from build123d import *


with BuildPart() as part:
    # Sketch1 → Revolve1 (revolve)
    with BuildSketch(Plane.XY, mode=Mode.PRIVATE) as revolve1_sk:
        with BuildLine():
            Line((-40, 20), (-50, 20))
            Line((-50, 20), (-50, 0))
            Line((-50, 0), (0, 0))
            Line((0, 0), (0, 12.26993865))
            Line((0, 12.26993865), (29.439071242, 12.26993865))
            Line((29.439071242, 12.26993865), (29.439071242, 28.82661238))
            Line((29.439071242, 28.82661238), (26.939071242, 28.82661238))
            Line((26.939071242, 28.82661238), (26.939071242, 70.956055766))
            ThreePointArc((26.939071242, 70.956055766), (25.684040418, 70.638264837), (24.439071242, 70.283095588))
            Line((24.439071242, 70.283095588), (24.439071242, 28.82661238))
            Line((24.439071242, 28.82661238), (19.439071242, 28.82661238))
            Line((19.439071242, 28.82661238), (19.439071242, 68.432672522))
            ThreePointArc((19.439071242, 68.432672522), (18.179445476, 67.85181502), (16.939071242, 67.230909015))
            Line((16.939071242, 67.230909015), (16.939071242, 28.82661238))
            Line((16.939071242, 28.82661238), (11.939071242, 28.82661238))
            Line((11.939071242, 28.82661238), (11.939071242, 64.18039577))
            ThreePointArc((11.939071242, 64.18039577), (10.671746733, 63.249245387), (9.439071242, 62.272688383))
            Line((9.439071242, 62.272688383), (9.439071242, 28.82661238))
            Line((9.439071242, 28.82661238), (4.439071242, 28.82661238))
            Line((4.439071242, 28.82661238), (4.439071242, 52.883509313))
            Line((4.439071242, 52.883509313), (-10.560928758, 52.883509313))
            Line((-10.560928758, 52.883509313), (-25.483605064, 42.81803705))
            Line((-25.483605064, 42.81803705), (-25.483605064, 26.193767786))
            Line((-25.483605064, 26.193767786), (-25.483605064, 21.51803705))
            Line((-25.483605064, 21.51803705), (-25.483605064, 21.193767786))
            Line((-25.483605064, 21.193767786), (-25.483605064, 20))
            ThreePointArc((-25.483605064, 20), (-28.412537252, 12.928932188), (-35.483605064, 10))
            Line((-35.483605064, 10), (-40, 10))
            Line((-40, 10), (-40, 20))
        make_face()
        with BuildLine():
            Line((29.439071242, 28.82661238), (29.439071242, 12.26993865))
            Line((29.439071242, 12.26993865), (44.439071242, 12.26993865))
            Line((44.439071242, 12.26993865), (44.439071242, 28.82661238))
            Line((44.439071242, 28.82661238), (41.939071242, 28.82661238))
            Line((41.939071242, 28.82661238), (41.939071242, 71.836959972))
            ThreePointArc((41.939071242, 71.836959972), (40.690646644, 71.963785236), (39.439071242, 72.054381233))
            Line((39.439071242, 72.054381233), (39.439071242, 28.82661238))
            Line((39.439071242, 28.82661238), (34.439071242, 28.82661238))
            Line((34.439071242, 28.82661238), (34.439071242, 72.054381233))
            ThreePointArc((34.439071242, 72.054381233), (33.187495839, 71.963785236), (31.939071242, 71.836959972))
            Line((31.939071242, 71.836959972), (31.939071242, 28.82661238))
            Line((31.939071242, 28.82661238), (29.439071242, 28.82661238))
        make_face()
        with BuildLine():
            Line((44.439071242, 28.82661238), (44.439071242, 12.26993865))
            Line((44.439071242, 12.26993865), (100, 12.26993865))
            Line((100, 12.26993865), (100, 27.26993865))
            Line((100, 27.26993865), (80, 27.26993865))
            Line((80, 27.26993865), (80, 48.56993865))
            Line((80, 48.56993865), (70, 48.56993865))
            Line((70, 48.56993865), (70, 28.82661238))
            Line((70, 28.82661238), (65, 28.82661238))
            Line((65, 28.82661238), (65, 61.803487266))
            ThreePointArc((65, 61.803487266), (63.768152096, 62.813233579), (62.5, 63.776990361))
            Line((62.5, 63.776990361), (62.5, 28.82661238))
            Line((62.5, 28.82661238), (56.939071242, 28.82661238))
            Line((56.939071242, 28.82661238), (56.939071242, 67.230909015))
            ThreePointArc((56.939071242, 67.230909015), (55.698697008, 67.85181502), (54.439071242, 68.432672522))
            Line((54.439071242, 68.432672522), (54.439071242, 28.82661238))
            Line((54.439071242, 28.82661238), (49.439071242, 28.82661238))
            Line((49.439071242, 28.82661238), (49.439071242, 70.283095588))
            ThreePointArc((49.439071242, 70.283095588), (48.194102066, 70.638264837), (46.939071242, 70.956055766))
            Line((46.939071242, 70.956055766), (46.939071242, 28.82661238))
            Line((46.939071242, 28.82661238), (44.439071242, 28.82661238))
        make_face()
    revolve(revolve1_sk.sketch.rotate(Axis((-50, -15, 0), (1, 0, 0)), 180), axis=Axis((-50, -15, 0), (1, 0, 0)))


solid = part.part
Can you work these out from the model? Positions are in its coordinate system, mm. A direction names the side the tool comes from. Coordinates: 2 decimals unless noted, no trailing zeros. Order: outer loops, then holes, each group sorted by start corner. A loop starts at its lowest first (then second) coordinate and runs counter-clockwise, first axis right, second up. Notation, with made-up numbers: (87.5, 87.5) - (114.5, 87.5) arc R14 ccw to (114.5, 94.5) - close; hole circle Ø5 at (86.5, 79.5). An arc over 180 degrees is marked (long way). Answer as a JSON object with one key per item and string values. Group by question number.
Q1. Imagine slicing it at A-A (x = -3). Please give me the cut outline in (y, z), and give its area (3 significant figures).
Q2. Imagine slicing it at D-D (x = 22). Please give me the cut outline in (y, z), and give its area (3 significant figures).
Q3. I need wall thicknesses on line 1 (X direction, y = -92.5, z = -22.5); line 2 (Z direction, x = -36.5, y = -15); line 3 (Z direction, x = -17, y = -15). Which ranges of each line are inside material? Lowest first, please. Write a range as from..to.
Q4. Will these pins go through, and if not, where does the flat tip stop? P1, Ø10, axis at y = 32.5, z = 18, coming from the -X side; P2, Ø6, axis at x = -12, y = 25.5, coming from the +Z side; P3, Ø12, axis at x = 63, z = -51, coming from the +Y side.
Q5. We'd pull the mould along X, two halves only. Please class faces 1 (the face through (80, -2, 41)), 2 (the face through (4.439, -16, 44)), 3 (the face through (-50, -30, 7)): +X half, -X half, draft (parallel to the pull), parting line (faces both ways), or undercut.
Q6. Imagine slicing it at B-B (z = -72). Give the number of separate pieces and of enclosed holes in the cut face, and give its area (3 significant figures).
Q7. On a 3-axis mill with a long thin cutter (end or side, diameter ignored), from which of +Z, -Z, +X, -X, +Y, -Y can I reach the whole of each face in a straight line? I mean faces 4 (the face through (50.7, -11.45, -27.038)), 5 (the face through (-45.07, -7.413, 34.168)), 6 (the face through (21.904, -9.295, -43.454)), 7 (the face through (-24.65, -0.015, -0.66)). Say none if no direction works.
Determined:
{
 "1": {"outline": "circle Ø135.77 at (-15, 0); hole circle Ø30 at (-15, 0)", "area": "13,800 mm2"},
 "2": {"outline": "circle Ø87.65 at (-15, 0); hole circle Ø54.54 at (-15, 0)", "area": "3,700 mm2"},
 "3": {"line 1": "x = 16.94..19.44, 24.44..26.94, 31.94..34.44, 39.44..41.94, 46.94..49.44, 54.44..56.94", "line 2": "z = -25..-15, 15..25", "line 3": "z = -63.54..-15, 15..63.54"},
 "4": {"P1": "stops at x = -25.48", "P2": "stops at z = 56.34", "P3": "stops at y = 49.64"},
 "5": {"face 1": "+X half", "face 2": "undercut", "face 3": "-X half"},
 "6": {"separate pieces": "8", "enclosed holes": "0", "area": "1,660 mm2"},
 "7": {"face 4": "+X", "face 5": "-X", "face 6": "none", "face 7": "+X, -X"}
}
